The listing builds one solid part. Answer for the finished solid, in the listing's coordinates (mm). A direction names the side the tool comes from. Give positions to 0.01 mm unless a question says otherwise; leave off trailing zeros. Loops run counter-clockwise (first coordinate to the right, second up) from the corner with the lowest first, then second, coordinate; pieces in that order, holes last. Notation, with made-up numbers: (-30.5, 19.25) - (-23.5, 19.25) arc R25 cw to (-23.5, 34.25) - close; hole circle Ø11 at (80, -10). An arc over 180 degrees is marked (long way). Write each question's results on one line, items separated by ' | '.
from build123d import *

# Parameters (mm, degrees)
CYLINDER106_R     = 1.5
CYLINDER106_DEPTH = 108
CYLINDER105_R     = 5.5
CYLINDER105_DEPTH = 60
CYLINDER108_R     = 9.5
CYLINDER108_DEPTH = 3


with BuildPart() as obj1:
    # Cylinder106 → Cylinder106 (new body)
    with BuildSketch(Plane(origin=(86.69, 175.69, -20), x_dir=(1, 0, 0), z_dir=(0, 0, 1))):
        Circle(CYLINDER106_R)
    extrude(amount=CYLINDER106_DEPTH)


with BuildPart() as obj2:
    # Cylinder105 → Cylinder105 (new body)
    with BuildSketch(Plane(origin=(86.69, 175.69, -16), x_dir=(1, 0, 0), z_dir=(0, 0, 1))):
        Circle(CYLINDER105_R)
    extrude(amount=CYLINDER105_DEPTH)


with BuildPart() as obj3:
    # Cylinder108 → Cylinder108 (new body)
    with BuildSketch(Plane(origin=(86.69, 175.69, -8), x_dir=(1, 0, 0), z_dir=(0, 0, 1))):
        Circle(CYLINDER108_R)
    extrude(amount=CYLINDER108_DEPTH)

    # Fusion044: union obj2
    add(obj2.part)

    # Cut012: cut obj1
    add(obj1.part, mode=Mode.SUBTRACT)


solid = obj3.part
Item 1: A cutting plane is placed at A-A, the plane y = 175.69. Determine the outline of the cut face in (x, z), plus the area to 3 significant figures.
Values found:
outline: (77.19, -8) - (81.19, -8) - (81.19, -16) - (85.19, -16) - (85.19, 44) - (81.19, 44) - (81.19, -5) - (77.19, -5) - close; (88.19, -16) - (92.19, -16) - (92.19, -8) - (96.19, -8) - (96.19, -5) - (92.19, -5) - (92.19, 44) - (88.19, 44) - close | area: 504 mm²
Item 2: For a pull along Y with two mould halves and no side action, classify faces 4 (the face through (89.23, 170.81, 19.16)), 5 (the face through (86.495, 177.177, 13.58)), 6 (the face through (85, 175, -16)) as released by +Y, released by -Y, zero draft, split by the parting line, or undercut.
Values found:
face 4: split by the parting line | face 5: undercut | face 6: zero draft
Item 3: A cutting plane is placed at D-D, the plane y = 170.75. Determine the outline of the cut face in (x, z).
Values found:
outline: (78.58, -8) - (84.27, -8) - (84.27, -16) - (89.11, -16) - (89.11, -8) - (94.8, -8) - (94.8, -5) - (89.11, -5) - (89.11, 44) - (84.27, 44) - (84.27, -5) - (78.58, -5) - close
Item 4: Flat-ended cylindrical pins translate along their axes: P1, Ø5, axis at y = 181, z = 0.5, coming from the +X side; P2, Ø4, axis at x = 92, z = -3.5, coming from the -Y side; P3, Ø5, axis at y = 173.5, z = 17, coming from the -X side. Find the tip coordinate at first contact, or state that the pin passes through.
Values found:
P1: stops at x = 91.42 | P2: stops at y = 167.07 | P3: stops at x = 81.19
Item 5: Find the intervals of material crossed by line 1 along Y through (x, z) = (86.69, 12); line 2 along X through (y, z) = (175.5, 3.5); line 3 along Z through (x, y) = (85, 182.25), in increasing order. Write a range as [from, to].
Values found:
line 1: y = [170.19, 174.19], [177.19, 181.19] | line 2: x = [81.19, 85.2], [88.18, 92.19] | line 3: z = [-8, -5]
Item 6: A cutting plane is placed at C-C, the plane z = 8.5. Determine the outline of the cut face in (x, y).
Values found:
outline: circle Ø11 at (86.69, 175.69); hole circle Ø3 at (86.69, 175.69)
Item 7: For faces 1 (the face through (89.23, 170.81, -12.06)), 2 (the face through (91, 172, -5)), 3 (the face through (85, 175, 44)), determine the directions among +Z, -Z, +X, -X, +Y, -Y from which every point of the face is accessible in a straight line to the end or side of a thin tool.
Values found:
face 1: -Z | face 2: +Z | face 3: +Z, +X, -X, +Y, -Y
Item 8: A cutting plane is placed at B-B, the plane x = 84.5. Determine the outline of the cut face in (y, z).
Values found:
outline: (166.45, -8) - (170.64, -8) - (170.64, -16) - (180.74, -16) - (180.74, -8) - (184.93, -8) - (184.93, -5) - (180.74, -5) - (180.74, 44) - (170.64, 44) - (170.64, -5) - (166.45, -5) - close
